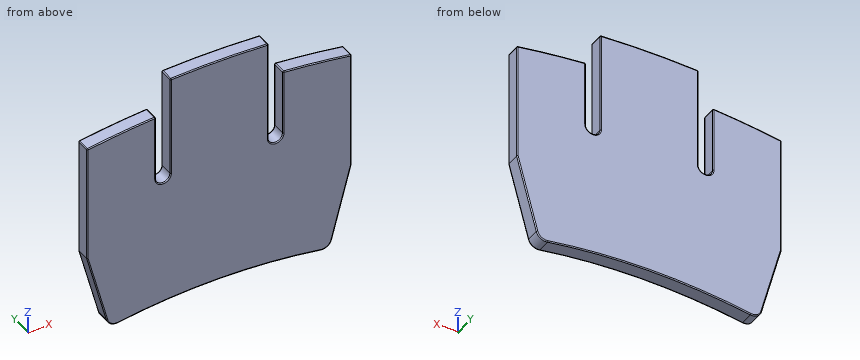
from build123d import *

# Parameters (mm, degrees)
BOSS_EXTRUDE1_DEPTH = 3
FILLET1_R           = 0.2


with BuildPart() as part:
    # Sketch1 → Boss-Extrude1 (new body)
    with BuildSketch(Plane(origin=(0, 0, 0), x_dir=(1, 0, 0), z_dir=(0, 1, 0))):
        with BuildLine():
            Line((-10, 29), (-10, 8.285947903))
            ThreePointArc((-10, 8.285947903), (0, 8), (10, 8.285947903))
            Line((10, 8.285947903), (10, 29))
            ThreePointArc((10, 29), (11.5, 30.5), (13, 29))
            Line((13, 29), (13, 15.503731385))
            ThreePointArc((13, 15.503731385), (20.017634438, 16.196839624), (27, 17.183836735))
            Line((27, 17.183836735), (27, 41.21477169))
            Line((27, 41.21477169), (22.972622015, 56.245150951))
            ThreePointArc((22.972622015, 56.245150951), (22.124373546, 57.408525693), (20.714556868, 57.700729716))
            ThreePointArc((20.714556868, 57.700729716), (0, 56), (-20.714556868, 57.700729716))
            ThreePointArc((-20.714556868, 57.700729716), (-22.124373546, 57.408525693), (-22.972622015, 56.245150951))
            Line((-22.972622015, 56.245150951), (-27, 41.21477169))
            Line((-27, 41.21477169), (-27, 17.183836735))
            ThreePointArc((-27, 17.183836735), (-20.017634438, 16.196839624), (-13, 15.503731385))
            Line((-13, 15.503731385), (-13, 28.994346903))
            ThreePointArc((-13, 28.994346903), (-11.50283188, 30.500002663), (-10, 29))
        make_face()
    extrude(amount=BOSS_EXTRUDE1_DEPTH)

    # Fillet1
    fillet1_edges = [part.edges().sort_by_distance(p)[0] for p in [
        (0, 3, -8),
        (10, 3, -18.642973952),
        (-13, 0, -22.249039144),
        (-20.017634438, 0, -16.196839624),
        (-27, 0, -29.199304212),
        (-24.986311008, 0, -48.729961321),
        (-22.124373546, 0, -57.408525693),
        (11.5, 3, -30.5),
        (0, 0, -56),
        (22.124373546, 0, -57.408525693),
        (24.986311008, 0, -48.729961321),
        (27, 0, -29.199304212),
        (20.017634438, 0, -16.196839624),
        (13, 0, -22.251865692),
        (11.5, 0, -30.5),
        (10, 0, -18.642973952),
        (13, 3, -22.251865692),
        (0, 0, -8),
        (-10, 0, -18.642973952),
        (-11.50283188, 0, -30.500002663),
        (20.017634438, 3, -16.196839624),
        (27, 3, -29.199304212),
        (-13, 1.5, -15.503731385),
        (-27, 1.5, -17.183836735),
        (27, 1.5, -17.183836735),
        (13, 1.5, -15.503731385),
        (10, 1.5, -8.285947903),
        (-10, 1.5, -8.285947903),
        (24.986311008, 3, -48.729961321),
        (22.124373546, 3, -57.408525693),
        (0, 3, -56),
        (-22.124373546, 3, -57.408525693),
        (-11.50283188, 3, -30.500002663),
        (-24.986311008, 3, -48.729961321),
        (-27, 3, -29.199304212),
        (-20.017634438, 3, -16.196839624),
        (-13, 3, -22.249039144),
        (-10, 3, -18.642973952),
    ]]
    fillet(fillet1_edges, radius=FILLET1_R)


solid = part.part
Input: part model. Units: mm. Frame: model coordinates. Give positions to 0.01 mm unless a question says otherwise; leave off trailing zeros. Loops run counter-clockwise (first coordinate to the right, second up) from the corner with the lowest first, then second, coordinate; pieces in that order, holes last. Notation, with made-up numbers: (22, -37.5) -> (33, -37.5) arc R18 ccw to (33, -8.5) -> close; hole circle Ø2 at (32.5, -20). An arc over 180 degrees is marked (long way). Answer as a JSON object with one key per item and string values. Group by question number.
Item 1: Pin query (flat end, axial travel): P1, Ø5, axis at x = 19.5, z = -23, coming from the -Y side; P2, Ø1.5, axis at x = 2.5, y = 1, coming from the -Z side. Return the tip coordinate at first contact, or that it passes through.
Item 2: Line query: probe 1 along X at (y, z) = (0.85, -25.5); probe 2 along X at (y, z) = (1.45, -14); probe 3 along X at (y, z) = (2.2, -29.5). Output: solid intervals per line, ascending.
Item 3: Cut plane B-B, the plane y = 1.6. Return the cut outline in (x, z), and give its area (3 significant figures).
Item 4: Cut plane A-A, the plane z = -24.5. Return the cut outline in (x, y).
Checks:
{
 "1": {"P1": "stops at y = 0", "P2": "stops at z = -56.04"},
 "2": {"probe 1": "x = -27 to -13, -10 to 10, 13 to 27", "probe 2": "x = -10 to 10", "probe 3": "x = -27 to -12.91, -10.09 to 10.09, 12.91 to 27"},
 "3": {"outline": "(-27, -41.21) -> (-22.97, -56.25) arc R2 ccw to (-20.71, -57.7) arc R127 cw to (20.71, -57.7) arc R2 ccw to (22.97, -56.25) -> (27, -41.21) -> (27, -17.35) arc R0.2 ccw to (26.83, -17.16) arc R168 ccw to (13.22, -15.52) arc R0.2 ccw to (13, -15.72) -> (13, -29) arc R1.5 cw to (10, -29) -> (10, -8.47) arc R0.2 ccw to (9.81, -8.28) arc R175 ccw to (-9.81, -8.28) arc R0.2 ccw to (-10, -8.47) -> (-10, -29) arc R1.5 cw to (-13, -28.99) -> (-13, -15.72) arc R0.2 ccw to (-13.22, -15.52) arc R168 ccw to (-26.83, -17.16) arc R0.2 ccw to (-27, -17.35) -> close", "area": "2,200 mm²"},
 "4": {"outline": "(-27, 0.2) arc R0.2 ccw to (-26.8, 0) -> (-13.2, 0) arc R0.2 ccw to (-13, 0.2) -> (-13, 2.8) arc R0.2 ccw to (-13.2, 3) -> (-26.8, 3) arc R0.2 ccw to (-27, 2.8) -> close; (-10, 0.2) arc R0.2 ccw to (-9.8, 0) -> (9.8, 0) arc R0.2 ccw to (10, 0.2) -> (10, 2.8) arc R0.2 ccw to (9.8, 3) -> (-9.8, 3) arc R0.2 ccw to (-10, 2.8) -> close; (13, 0.2) arc R0.2 ccw to (13.2, 0) -> (26.8, 0) arc R0.2 ccw to (27, 0.2) -> (27, 2.8) arc R0.2 ccw to (26.8, 3) -> (13.2, 3) arc R0.2 ccw to (13, 2.8) -> close"}
}
